Autodesk Inventor part; units mm, degrees
ref_plane "YZ Plane" through (0, 0, 0) normal (1, 0, 0) x (0, 1, 0)
ref_plane "XZ Plane" through (0, 0, 0) normal (0, 1, 0) x (-1, 0, 0)
ref_plane "XY Plane" through (0, 0, 0) normal (0, 0, 1) x (1, 0, 0)
sketch "Sketch1" plane through (0, 0, 0) normal (0, 0, 1) x (1, 0, 0)
  line L0 (14.1765, -19.066) -> (14.1765, 161.6208)
  line L1 (14.1765, -19.066) -> (79.1765, -19.066)
  line L2 (79.1765, -19.066) -> (79.1765, 155.934)
  line L3 (79.1765, -19.066) -> (14.1765, -19.066)
  line L4 (79.1765, -19.066) -> (14.1765, -19.066)
  line L5 (14.1765, 161.6208) -> (79.1765, 155.934)
  line L6 (79.1765, 135.934) -> (74.1765, 135.934)
  line L7 (74.1765, 135.934) -> (74.1765, 115.934)
  line L8 (74.1765, 115.934) -> (79.1765, 115.934)
  line L9 (79.1765, 115.934) -> (79.1765, 135.934)
  line L10 (69.1765, 20.934) -> (74.1765, 20.934)
  line L11 (74.1765, 20.934) -> (74.1765, 0.934)
  line L12 (74.1765, 0.934) -> (69.1765, 0.934)
  line L13 (69.1765, 0.934) -> (69.1765, 20.934)
  line L14 (74.1765, 135.934) -> (69.1765, 135.934)
  line L15 (69.1765, 135.934) -> (69.1765, 115.934)
  line L16 (69.1765, 115.934) -> (74.1765, 115.934)
  line L17 (74.1765, 115.934) -> (74.1765, 135.934)
  point P0 (0, 0)
  point P1 (71.6765, 0.934)
  point P2 (79.2985, 0.69)
  point P3 (79.2985, 20.69)
  point P4 (79.1765, 115.934)
  dimension "d3" = 65
  dimension "d23" = 85
  dimension "d26" = 175
  dimension "d27" = 180.6868
  dimension "d28" = 5
  dimension "d29" = 20
  dimension "d30" = 5
  dimension "d31" = 20
  dimension "d32" = 20
  dimension "d33" = 20
  dimension "d35" = 5
  dimension "d36" = 5
extrude "Extrusion1" add sketch "Sketch1" along normal mid plane 5 contours L0 L5 L2 L6 L14 L15 L16 L8 L1 | L8 L7 L6 L2
equation "\"BendRadius\" = Thickness"
equation "\"BendReliefWidth\" = Thickness"
equation "\"BendReliefDepth\" = 0.5 * Thickness"
equation "\"CornerReliefSize\" = 4 * Thickness"
equation "\"MinimumRemnant\" = 2 * Thickness"
equation "\"TransitionRadius\" = BendRadius"
equation "\"JacobiRadiusSize\" = BendRadius"
equation "\"GapSize\" = Thickness"
properties part number "stand"
Input: part model. Units: mm. Frame: model coordinates. A direction names the side the tool comes from. Coordinates: 2 decimals unless noted, no trailing zeros. Loops run counter-clockwise (first coordinate to the right, second up) from the corner with the lowest first, then second, coordinate; pieces in that order, holes last. Notation, with made-up numbers: (-13, 74) - (33, 74) arc R33 cw to (33, 105) - close; hole circle Ø2 at (88, -21.75). An arc over 180 degrees is marked (long way). Answer in a Markdown table with one row per item. Add a question column.
Item 1: Section query B-B on x = 57.5. Return the cut outline in (y, z), then the cut area to 3 significant figures.
Item 2: Access query for faces 1 (the flat face through (46, 73, -2.5)), 2 (the flat face through (72, 20.934, 0)). Directions: +Z, -Z, +X, -X, +Y, -Y. A direction counts if a zero-diameter tool reaches every point of the face in a straight line with its end or side. Return the directions, or none.
Item 3: Section query C-C on x = 50.5. Return the cut outline in (y, z).
Item 4: Contact query for flat-ended pins moving along their axis: P1, Ø1, axis at x = 47, z = 2, coming from the +Y side; P2, Ø2.5, axis at x = 71.5, z = 0.5, coming from the +Y side (3 decimals). Output: stop coordinate, or through.
Item 5: Line query: line 1 along X through (y, z) = (14, 0.2); line 2 along Y through (x, z) = (70, -0.5); line 3 along Y through (x, z) = (75.5, -1.15). Output: solid intervals per line, ascending. Write a range as [from, to].
Item 6: Mould query, pull axis X, two halves, no side actions, for faces 3 (the flat face through (14.176, 70, 0)), 4 (the flat face through (46.221, 158.817, -0.035)), 5 (the flat face through (74.176, 11, 0)), 6 (the flat face through (72, 135.934, 0)). Classes: released by +X, released by -X, zero draft, split by the parting line, or undercut.
Item 7: Section query A-A on z = 0. Return the cut outline in (x, y), then the cut area to 3 significant figures.
Recorded:
| question | item | result |
|---|---|---|
| 1 | outline | (-19.07, -2.5) - (157.83, -2.5) - (157.83, 2.5) - (-19.07, 2.5) - close |
| 1 | area | 884 mm^2 |
| 2 | face 1 | -Z, +X, -X, +Y, -Y |
| 2 | face 2 | +Z, -Z |
| 3 | outline | (-19.07, -2.5) - (158.44, -2.5) - (158.44, 2.5) - (-19.07, 2.5) - close |
| 4 | P1 | y = 158.79 |
| 4 | P2 | y = 156.715 |
| 5 | line 1 | [14.18, 69.18], [74.18, 79.18] |
| 5 | line 2 | [-19.07, 0.93], [20.93, 115.93], [135.93, 156.74] |
| 5 | line 3 | [-19.07, 156.26] |
| 6 | face 3 | released by -X |
| 6 | face 4 | released by +X |
| 6 | face 5 | undercut |
| 6 | face 6 | undercut |
| 7 | outline | (14.18, -19.07) - (79.18, -19.07) - (79.18, 155.93) - (14.18, 161.62) - close; hole (69.18, 0.93) - (74.18, 0.93) - (74.18, 20.93) - (69.18, 20.93) - close; hole (69.18, 115.93) - (74.18, 115.93) - (74.18, 135.93) - (69.18, 135.93) - close |
| 7 | area | 11,400 mm^2 |
